Could you check a few things on this model? Use its own coordinates, in mm. A direction names the side the tool comes from. Round coordinates to 2 decimals unless told otherwise and drop trailing zeros. Write each loop counter-clockwise with the first axis right and the second up, starting at its lowest first coordinate (ties: lowest second). Pieces come first, ordered by that corner, then holes. Notation, with made-up numbers: M 22,51 L 47,51 A24 cw 47,64 Z; hole C 4,52 d6. An arc over 180 degrees is marked long. One line per item, written item: value. Start each with the question number.
(1) I want a section at A-A on y = 3.1. Please give me the cut outline in (x, z) (3 decimals), and give its area (3 significant figures).
(2) I want a section at D-D on x = 1.25. Please give me the cut outline in (y, z) (3 decimals), and give its area (3 significant figures).
(3) If I drill on L1, parallel to X at y = 1, z = 0 (3 decimals); L2, parallel to Z at x = 2, y = 4.25 (3 decimals); L3, parallel to X at y = 2, z = -6.11 (3 decimals), over which ranges is the centre line in solid material (lowest first)?
(4) I'm going to push flat-ended pins straight in: pin 1 Ø4 at (x, z) = (0, -6.11) entering from -Y; pin 2 Ø1 at (x, z) = (3.5, -9) entering from +Y. Where does each tip first touch, or does it pass through?
(5) Thinking about a two-plate mould opening in Y: for faces 4 (the face through (-2.78, 1.782, -0.072)), 5 (the face through (-3, 3, 2.325)), 6 (the face through (-0.3, 6.2, -2.6)), 7 (the face through (2.835, 1.782, -0.072)), which applies, released by +Y, released by -Y, zero draft, split by the parting line, or undercut?
(6) Which directions (+Z, -Z, +X, -X, +Y, -Y) give clear straight access to the entire face, cutting with the end or side of a thin tool? Please do faces 1 (the face through (-0.508, 6.446, -9.977)), 2 (the face through (0.128, 3.143, -9.282)), 3 (the face through (-0.85, 5, 0)).
(7) I want a section at C-C on z = -2. Please give me the cut outline in (x, y) (3 decimals), and give its area (3 significant figures).
(8) I want a section at B-B on x = 0. Please give me the cut outline in (y, z) (3 decimals), and give its area (3 significant figures).
```python
from build123d import *

# Parameters (mm, degrees)
CROQUIS1_R              = 4.765
CROQUIS1_W              = 9.53
CROQUIS1_H              = 4.65
SALIENTE_EXTRUIR1_DEPTH = 6.2
CROQUIS2_R              = 3.175
CORTAR_EXTRUIR1_DEPTH   = 6.2
CROQUIS3_W              = 1.7
CROQUIS3_H              = 5.8
CORTAR_EXTRUIR2_DEPTH   = 6.2
CROQUIS4_R              = 1.35
CORTAR_EXTRUIR3_DEPTH   = 10.53
CROQUIS5_R              = 3.9
SALIENTE_EXTRUIR2_DEPTH = 0.5
CROQUIS6_R              = 3.15
CORTAR_EXTRUIR4_DEPTH   = 7.7


with BuildPart() as part:
    # Croquis1 → Saliente-Extruir1 (new body)
    with BuildSketch(Plane(origin=(0, 0, 0), x_dir=(1, 0, 0), z_dir=(0, 1, 0))):
        with Locations((0, 6.11)):
            Circle(CROQUIS1_R)
        Rectangle(CROQUIS1_W, CROQUIS1_H)
        with BuildLine():
            ThreePointArc((4.765, 6.11), (0, 10.875), (-4.765, 6.11))
            ThreePointArc((-4.765, 6.11), (-4.271898488, 3.999050378), (-2.894650238, 2.325))
            Line((-2.894650238, 2.325), (2.894650238, 2.325))
            ThreePointArc((2.894650238, 2.325), (4.271898488, 3.999050378), (4.765, 6.11))
        make_face()
        with BuildLine():
            Line((2.894650238, 2.325), (-2.894650238, 2.325))
            ThreePointArc((-2.894650238, 2.325), (0, 1.345), (2.894650238, 2.325))
        make_face()
        with BuildLine():
            Line((-4.765, 6.11), (-4.765, 2.325))
            Line((-4.765, 2.325), (-2.894650238, 2.325))
            ThreePointArc((-2.894650238, 2.325), (-4.271898488, 3.999050378), (-4.765, 6.11))
        make_face()
        with BuildLine():
            Line((4.765, 2.325), (4.765, 6.11))
            ThreePointArc((4.765, 6.11), (4.271898488, 3.999050378), (2.894650238, 2.325))
            Line((2.894650238, 2.325), (4.765, 2.325))
        make_face()
    extrude(amount=SALIENTE_EXTRUIR1_DEPTH)

    # Croquis2 → Cortar-Extruir1 (cut)
    with BuildSketch(Plane(origin=(0, 6.2, 0), x_dir=(1, 0, 0), z_dir=(0, 1, 0))):
        with Locations((0, 6.11)):
            Circle(CROQUIS2_R)
    extrude(amount=-CORTAR_EXTRUIR1_DEPTH, mode=Mode.SUBTRACT)

    # Croquis3 → Cortar-Extruir2 (cut)
    with BuildSketch(Plane(origin=(0, 6.2, 0), x_dir=(1, 0, 0), z_dir=(0, 1, 0))):
        with Locations((0, 0.575)):
            Rectangle(CROQUIS3_W, CROQUIS3_H)
    extrude(amount=-CORTAR_EXTRUIR2_DEPTH, mode=Mode.SUBTRACT)

    # Croquis4 → Cortar-Extruir3 (cut, through all)
    with BuildSketch(Plane(origin=(4.765, 0, 0), x_dir=(0, 0, -1), z_dir=(1, 0, 0))):
        with Locations((0.365, 3.1)):
            Circle(CROQUIS4_R)
    extrude(amount=-CORTAR_EXTRUIR3_DEPTH, mode=Mode.SUBTRACT)

    # Croquis5 → Saliente-Extruir2 (add)
    with BuildSketch(Plane(origin=(0, 6.2, 0), x_dir=(1, 0, 0), z_dir=(0, 1, 0))):
        with Locations((0, 6.11)):
            Circle(CROQUIS5_R)
    extrude(amount=SALIENTE_EXTRUIR2_DEPTH)

    # Croquis6 → Cortar-Extruir4 (cut, through all)
    with BuildSketch(Plane(origin=(0, 6.7, 0), x_dir=(1, 0, 0), z_dir=(0, 1, 0))):
        with Locations((0, 6.11)):
            Circle(CROQUIS6_R)
    extrude(amount=-CORTAR_EXTRUIR4_DEPTH, mode=Mode.SUBTRACT)


solid = part.part
```
Found:
1. outline: M -4.765,-6.11 A4.765 ccw 4.765,-6.11 L 4.765,-1.715 L 0.85,-1.715 L 0.85,-3.051 A3.175 cw long -0.85,-3.051 L -0.85,-1.715 L -4.765,-1.715 Z; M -4.765,0.985 L -0.85,0.985 L -0.85,2.325 L -4.765,2.325 Z; M 0.85,0.985 L 4.765,0.985 L 4.765,2.325 L 0.85,2.325 Z
1. area: 54.2 mm²
2. outline: M 0,-10.708 L 6.2,-10.708 L 6.2,-9.804 L 6.7,-9.804 L 6.7,-9.001 L 6.2,-9.001 L 6.2,-9.029 L 0,-9.029 Z; M 0,-3.191 L 6.2,-3.191 L 6.2,-3.219 L 6.7,-3.219 L 6.7,-2.416 L 6.2,-2.416 L 6.2,2.325 L 0,2.325 Z; hole C 3.1,-0.365 d2.7
2. area: 39.7 mm²
3. L1: x = -4.765 to -0.85, 0.85 to 4.765
3. L2: z = -10.435 to -8.576, -3.644 to -1.072, 0.342 to 2.325
3. L3: x = -4.765 to -3.175, 3.175 to 4.765
4. pin 1: passes through
4. pin 2: stops at y = 6.2
5. face 4: undercut
5. face 5: zero draft
5. face 6: released by -Y
5. face 7: undercut
6. face 1: +Y
6. face 2: -Y
6. face 3: +Z, -Y
7. outline: M -4.765,0 L -0.85,0 L -0.85,6.2 L -4.765,6.2 Z; M 0.85,0 L 4.765,0 L 4.765,6.2 L 0.85,6.2 Z
7. area: 48.5 mm²
8. outline: M 0,-10.875 L 6.2,-10.875 L 6.2,-10.01 L 6.7,-10.01 L 6.7,-9.26 L 6.2,-9.26 L 6.2,-9.285 L 0,-9.285 Z; M 6.2,-2.96 L 6.7,-2.96 L 6.7,-2.21 L 6.2,-2.21 Z
8. area: 10.6 mm²
